from build123d import *

# Parameters (mm, degrees)
SKETCH_1_R                = 62
SKETCH_1_R_2              = 44
EXTRUDE_373_DEPTH         = 5
PATTERN_CIRCULAR_M4_COUNT = 6


with BuildPart() as part:
    # Sketch 1 → Extrude 373 (new, symmetric)
    with BuildSketch(Plane(origin=(0, 0, 0), x_dir=(0, 0, -1), z_dir=(1, 0, 0))):
        Circle(SKETCH_1_R)
        Circle(SKETCH_1_R_2, mode=Mode.SUBTRACT)
    extrude(amount=EXTRUDE_373_DEPTH, both=True)

    # Sketch 2 → Hole Wizard M4 (revolve, cut)
    with BuildSketch(Plane(origin=(5, 54.25, 0), x_dir=(0, 0, -1), z_dir=(0, 1, 0))):
        Polygon((0, 0), (0, 11.351936393), (2.25, 10), (2.25, 0), align=None)
    hole_wizard_m4 = revolve(axis=Axis((11.35, 54.25, 0), (-1, 0, 0)), mode=Mode.SUBTRACT)

    # Pattern Circular M4: Hole Wizard M4 ×6 about axis
    pattern_circular_m4_axis = Axis((0, 0, 0), (1, 0, 0))
    for i in range(1, PATTERN_CIRCULAR_M4_COUNT):
        add(hole_wizard_m4.rotate(pattern_circular_m4_axis, i * 360 / PATTERN_CIRCULAR_M4_COUNT), mode=Mode.SUBTRACT)


solid = part.part
For this review, take the finished solid that the model builds, in its own axes (mm). Round coordinates to 2 decimals unless told otherwise and drop trailing zeros. Order: outer loops, then holes, each group sorted by start corner. A loop starts at its lowest first (then second) coordinate and runs counter-clockwise, first axis right, second up. Notation, with made-up numbers: M 81,57.5 L 127,57.5 A22 ccw 127,93.5 Z; hole C -34,-1 d6. An arc over 180 degrees is marked long. Write each question's results on one line, items separated by ' | '. Start each with the question number.
1. Add section D-D (x = 3). State the section outline as (y, z) points (3 decimals), then the cut area to 3 significant figures.
2. Add section C-C (z = -31.5). State the section outline as (x, y) points, then the cut area to 3 significant figures.
3. Add section A-A (z = 0). State the section outline as (x, y) points.
4. Add section B-B (y = 0). State the section outline as (x, z) points.
5. Clearance check with flat-ended pins moving along their axes: pin 1 Ø5 at (y, z) = (-27.12, 46.98) entering from -X; pin 2 Ø6 at (x, z) = (-3, 0) entering from -Y; pin 3 Ø4 at (x, z) = (-0.5, -13.5) entering from +Y; pin 4 Ø1.5 at (x, y) = (2, -11) entering from +Z. State where each tip first meets the part, or that it passes through.
6. Draft analysis for pull direction Z (two halves, no side actions). For faces 1 (the face through (5, 42, 15)), 2 (the face through (0.07, 26.26, 49.06)), 3 (the face through (0.07, 61.472, 8.071)), state which applies: pulls with the +Z half, pulls with the -Z half, needs draft (parallel to the pull), parting line crosses it, or undercut.
7. To check wall thickness, follow L1, parallel to Y at x = 2.25, z = 0; L2, parallel to Z at x = 1.5, y = -28; L3, parallel to Y at x = -4, z = 46. State the ranges of each line that lie inside material, in increasing order. Write a range as [from, to].
Output values:
1) outline: C 0,0 d124; hole C -54.25,0 d4.5; hole C 0,0 d88; hole C -27.125,-46.982 d4.5; hole C -27.125,46.982 d4.5; hole C 27.125,-46.982 d4.5; hole C 27.125,46.982 d4.5; hole C 54.25,0 d4.5 | area: 5,900 mm^2
2) outline: M -5,-53.4 L 5,-53.4 L 5,-30.72 L -5,-30.72 Z; M -5,30.72 L 5,30.72 L 5,53.4 L -5,53.4 Z | area: 454 mm^2
3) outline: M -5,-62 L 5,-62 L 5,-56.5 L -5,-56.5 Z; M -5,-52 L 5,-52 L 5,-44 L -5,-44 Z; M -5,44 L 5,44 L 5,52 L -5,52 Z; M -5,56.5 L 5,56.5 L 5,62 L -5,62 Z
4) outline: M -5,-62 L 5,-62 L 5,-44 L -5,-44 Z; M -5,44 L 5,44 L 5,62 L -5,62 Z
5) pin 1: x = -5 | pin 2: y = -62 | pin 3: y = 60.92 | pin 4: z = 61.15
6) face 1: needs draft | face 2: undercut | face 3: parting line crosses it
7) L1: [-62, -56.5], [-52, -44], [44, 52], [56.5, 62] | L2: [-55.32, -49.05], [-44.91, -33.94], [33.94, 44.91], [49.05, 55.32] | L3: [-41.57, -29.15], [-25.1, 25.1], [29.15, 41.57]
